```python
from build123d import *

# Parameters (mm, degrees)
SKETCH1_W           = 5.64
SKETCH1_H           = 18
BOSS_EXTRUDE1_DEPTH = 3
CUT_EXTRUDE1_START  = -4
CUT_EXTRUDE1_DEPTH  = 5


with BuildPart() as part:
    # Sketch1 → Boss-Extrude1 (new body)
    with BuildSketch(Plane(origin=(0, 0, 0), x_dir=(1, 0, 0), z_dir=(0, 1, 0))):
        Rectangle(SKETCH1_W, SKETCH1_H)
    extrude(amount=BOSS_EXTRUDE1_DEPTH)

    # Sketch2 → Cut-Extrude1 (cut)
    with BuildSketch(Plane(origin=(0, 3, 0), x_dir=(1, 0, 0), z_dir=(0, 1, 0)).offset(CUT_EXTRUDE1_START)):
        Polygon((-2.59, -9), (-2.59, -2), (-2.82, 2), (-2.82, -9), align=None)
    cut_extrude1 = extrude(amount=CUT_EXTRUDE1_DEPTH, mode=Mode.SUBTRACT)

    # Mirror1: Cut-Extrude1 across plane
    add(cut_extrude1.mirror(Plane(origin=(0, 0, 0), x_dir=(0, 0, 1), z_dir=(1, 0, 0))), mode=Mode.SUBTRACT)


solid = part.part
```
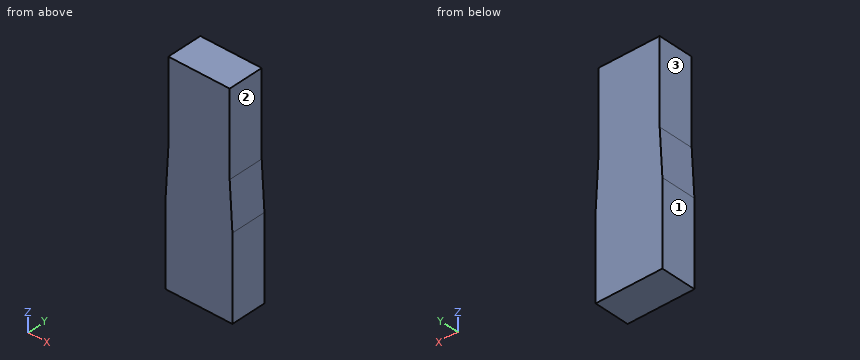
Work out the finished part from the listing and answer in its coordinate system (mm). Face numbers are marked on the shaded views. A direction names the side the tool comes from. Round coordinates to 2 decimals unless told otherwise and drop trailing zeros. Write each loop counter-clockwise with the first axis right and the second up, starting at its lowest first coordinate (ties: lowest second). Pieces come first, ordered by that corner, then holes.
1) Flat-ended cylindrical pins translate along their axes: P1, Ø1.5, axis at y = 2, z = 5, coming from the -X side; P2, Ø1.5, axis at y = 1, z = 5, coming from the +X side. Find the tip coordinate at first contact, or state that the pin passes through.
2) A cutting plane is placed at C-C on z = -1. Determine the outline of the cut face in (x, y), and give its area (3 significant figures).
3) Consider probe 1 along X at (y, z) = (0.75, 4.75). Determine where the line is inside the solid, lowest interval first.
4) Which of the six approach directions +Z, -Z, +X, -X, +Y, -Y give full straight-line access (tool end or side, diameter ignored) to the marked faces 1, 2 and 3?
5) A cutting plane is placed at A-A on y = 2.65. Determine the outline of the cut face in (x, z), and give its area (3 significant figures).
6) A cutting plane is placed at B-B on z = 5.5. Determine the outline of the cut face in (x, y), and give its area (3 significant figures).
Entries:
1. P1: stops at x = -2.59
1. P2: stops at x = 2.59
2. outline: (-2.76, 0) - (2.76, 0) - (2.76, 3) - (-2.76, 3) - close
2. area: 16.6 mm2
3. probe 1: x = -2.59 to 2.59
4. face 1: +Z, -Z, -X, +Y, -Y
4. face 2: +Z, +X, +Y, -Y
4. face 3: +Z, -X, +Y, -Y
5. outline: (-2.82, -9) - (2.82, -9) - (2.82, -2) - (2.59, 2) - (2.59, 9) - (-2.59, 9) - (-2.59, 2) - (-2.82, -2) - close
5. area: 97.4 mm2
6. outline: (-2.59, 0) - (2.59, 0) - (2.59, 3) - (-2.59, 3) - close
6. area: 15.5 mm2
